```python
from build123d import *

# Parameters (mm, degrees)
F0_R     = 1.719921
F1_DEPTH = 1.016
F0_R_2   = 5.863536
F0_R_3   = 0.379653
F2_DEPTH = 0.254
F3_DEPTH = 0.2794
F0_R_4   = 17.199212
F0_R_5   = 13.759369
F4_DEPTH = 1.27
F0_R_6   = 2.579882
F5_DEPTH = 0.127
F6_R     = 1.5875
F7_DEPTH = 25.4


with BuildPart() as f1:
    # F0 (on Front) → F1 (new body)
    with BuildSketch(Plane.XZ):
        with Locations((-22.672723, 24.880516)):
            Circle(F0_R)
    extrude(amount=F1_DEPTH)

    # F0 (on Front) → F2 (join)
    with BuildSketch(Plane.XZ):
        with Locations((-22.672723, 24.880516)):
            Circle(F0_R_2)
        with Locations((-23.476102, 20.220184)):
            Circle(F0_R_3, mode=Mode.SUBTRACT)
        with Locations((-26.53615, 22.153239)):
            Circle(F0_R_3, mode=Mode.SUBTRACT)
        with Locations((-19.945446, 21.017089)):
            Circle(F0_R_3, mode=Mode.SUBTRACT)
        with Locations((-18.012391, 24.077137)):
            Circle(F0_R_3, mode=Mode.SUBTRACT)
        with Locations((-27.333055, 25.683896)):
            Circle(F0_R_3, mode=Mode.SUBTRACT)
        with Locations((-25.4, 28.743944)):
            Circle(F0_R_3, mode=Mode.SUBTRACT)
        with Locations((-22.672723, 24.880516)):
            Circle(F0_R, mode=Mode.SUBTRACT)
        with Locations((-18.809295, 27.607794)):
            Circle(F0_R_3, mode=Mode.SUBTRACT)
        with Locations((-21.869343, 29.540849)):
            Circle(F0_R_3, mode=Mode.SUBTRACT)
    extrude(amount=F2_DEPTH)

    # F0 (on Front) → F3 (join)
    with BuildSketch(Plane.XZ):
        with Locations((-23.476102, 20.220184)):
            Circle(F0_R_3)
        with Locations((-19.945446, 21.017089)):
            Circle(F0_R_3)
        with Locations((-18.012391, 24.077137)):
            Circle(F0_R_3)
        with Locations((-18.809295, 27.607794)):
            Circle(F0_R_3)
        with Locations((-21.869343, 29.540849)):
            Circle(F0_R_3)
        with Locations((-25.4, 28.743944)):
            Circle(F0_R_3)
        with Locations((-27.333055, 25.683896)):
            Circle(F0_R_3)
        with Locations((-26.53615, 22.153239)):
            Circle(F0_R_3)
    extrude(amount=F3_DEPTH)



with BuildPart() as f4:
    # F0 (on Front) → F4 (new body, symmetric)
    with BuildSketch(Plane.XZ):
        with Locations((-22.672723, 24.880516)):
            Circle(F0_R_4)
        with Locations((-22.672723, 24.880516)):
            Circle(F0_R_5, mode=Mode.SUBTRACT)
    extrude(amount=F4_DEPTH, both=True)


with BuildPart() as f1_1:
    add(f1.part)

    add(f4.part)  # F5 merges F4
    # F0 (on Front) → F5 (join, symmetric)
    with BuildSketch(Plane.XZ):
        with Locations((-22.672723, 24.880516)):
            Circle(F0_R_5)
        with Locations((-27.788418, 15.907869)):
            Circle(F0_R_6, mode=Mode.SUBTRACT)
        with Locations((-32.634685, 22.153239)):
            Circle(F0_R_6, mode=Mode.SUBTRACT)
        with Locations((-19.945446, 14.918554)):
            Circle(F0_R_6, mode=Mode.SUBTRACT)
        with Locations((-13.700075, 19.764821)):
            Circle(F0_R_6, mode=Mode.SUBTRACT)
        with Locations((-31.64537, 29.996211)):
            Circle(F0_R_6, mode=Mode.SUBTRACT)
        with Locations((-25.4, 34.842479)):
            Circle(F0_R_6, mode=Mode.SUBTRACT)
        with Locations((-22.672723, 24.880516)):
            Circle(F0_R_2, mode=Mode.SUBTRACT)
        with Locations((-12.71076, 27.607794)):
            Circle(F0_R_6, mode=Mode.SUBTRACT)
        with Locations((-17.557028, 33.853164)):
            Circle(F0_R_6, mode=Mode.SUBTRACT)
    extrude(amount=F5_DEPTH, both=True)

    # F6 (on face) → F7 (cut)
    with BuildSketch(Plane.XZ.offset(1.016)):
        with Locations((-22.672723, 24.880516)):
            Circle(F6_R)
    extrude(amount=-F7_DEPTH, mode=Mode.SUBTRACT)


solid = f1_1.part
```
For this review, take the finished solid that the model builds, in its own axes (mm). A direction names the side the tool comes from. Round coordinates to 2 decimals unless told otherwise and drop trailing zeros. Write each loop counter-clockwise with the first axis right and the second up, starting at its lowest first coordinate (ties: lowest second). Pieces come first, ordered by that corner, then holes. Notation, with made-up numbers: (45.5, 42) - (64.5, 42) arc R21 ccw to (64.5, 49) - close; hole circle Ø4 at (-26, 22.25). An arc over 180 degrees is marked (long way). Answer as CSV lines item,"result". Start each with the question number.
(1) Add section A-A, the plane z = 35.5. State the section outline as (x, y) points, plus the area to 3 significant figures.
(2) For line 1 (X direction, y = 0.2, z = 36.5); line 2 (Z direction, x = -34, y = -0.9); line 3 (X direction, y = 0.65, z = 22), list the stretches that pass through material, from the lowest coordinate up.
(3) For pin 1 (4 mm diameter, centred on x = -25.4, z = 34.84, fed in from +Y) (3 decimals); pin 2 (3.5 mm diameter, centred on x = -23.5, z = 22.5, fed in from -Y); pin 3 (16.5 mm diameter, centred on x = -22.67, z = 24.88, fed in from +Y); pin 4 (0.6 mm diameter, centred on x = -22, z = 29.5, fed in from -Y), all flat-tipped, find the tip position at first contact; note any pin that passes through.
(4) Add section B-B, the plane x = -9.5. State the section outline as (y, z) points.
(5) Mouldability with a two-part tool opening along X and no side actions: class faces 4 (the flat face through (-18, 1.27, 38)), 5 (the flat face through (-21, 0, 24)), 6 (the cylindrical face through (-39.855, -0.018, 25.637)), 7 (the cylindrical face through (-25.66, -0.69, 11.45)) as +X half, -X half, draft (parallel to the pull), parting line (faces both ways), or undercut.
(6) Machinability: for faces 1 (the flat face through (-20, 0.127, 19)), 2 (the flat face through (-18, -1.27, 38)), 3 (the flat face through (-21, -0.254, 24)), which of the approach directions +Z, -Z, +X, -X, +Y, -Y give a long, thin tool a straight path to every point of the face, cutting with its end or side? Answer none if there is none.
From the geometry:
1,outline,"(-36.2, -1.27) - (-31.42, -1.27) - (-31.42, -0.13) - (-27.89, -0.13) - (-27.89, 0.13) - (-31.42, 0.13) - (-31.42, 1.27) - (-36.2, 1.27) - close; (-22.91, -0.13) - (-19.54, -0.13) - (-19.54, 0.13) - (-22.91, 0.13) - close; (-15.57, -0.13) - (-13.92, -0.13) - (-13.92, -1.27) - (-9.14, -1.27) - (-9.14, 1.27) - (-13.92, 1.27) - (-13.92, 0.13) - (-15.57, 0.13) - close"
1,area,"26.5 mm²"
2,line 1,"x = -35.35 to -30.04, -15.3 to -9.99"
2,line 2,"z = 11.94 to 17.07, 32.69 to 37.82"
2,line 3,"x = -39.63 to -36.13, -9.22 to -5.72"
3,pin 1,"passes through"
3,pin 2,"stops at y = -1.02"
3,pin 3,"stops at y = 0.13"
3,pin 4,"stops at y = -0.28"
4,outline,"(-1.27, 13.82) - (1.27, 13.82) - (1.27, 20.91) - (0.13, 20.91) - (0.13, 28.86) - (1.27, 28.86) - (1.27, 35.94) - (-1.27, 35.94) - (-1.27, 28.86) - (-0.13, 28.86) - (-0.13, 20.91) - (-1.27, 20.91) - close"
5,face 4,"draft"
5,face 5,"undercut"
5,face 6,"parting line"
5,face 7,"undercut"
6,face 1,"+Y"
6,face 2,"+Z, -Z, +X, -X, -Y"
6,face 3,"-Y"
